Read the model definition and answer for the solid it produces. Units are mm, in the model's axes. Face numbers are marked on the shaded views. A direction names the side the tool comes from. Round coordinates to 2 decimals unless told otherwise and drop trailing zeros. Write each loop counter-clockwise with the first axis right and the second up, starting at its lowest first coordinate (ties: lowest second). Pieces come first, ordered by that corner, then holes.
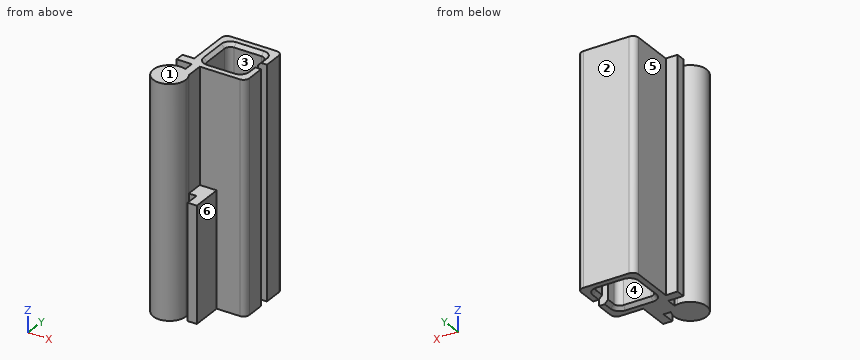
from build123d import *

# Parameters (mm, degrees)
F0_W     = 2.05
F0_H     = 1.6
F1_DEPTH = 40
F2_DEPTH = 20
F3_R     = 1
F4_SIZE  = 0.6


with BuildPart() as f1:
    # F0 (on Top) → F1 (new body)
    with BuildSketch(Plane.XY):
        Polygon((0.45, 6), (0.45, 4.4), (1.05, 4.4), (2.45, 4.4), (3.8, 4.4), (5.4, 4.4), (10.45, 4.4), (10.45, 8.6023478262), (8.85, 8.6023478262), (8.85, 6), (2.05, 6), (2.05, 12.8), (8.85, 12.8), (8.85, 10.1976521738), (10.45, 10.1976521738), (10.45, 14.4), (0.45, 14.4), align=None)
        with BuildLine():
            Line((2.45, 1.4), (2.45, 1.4560219779))
            ThreePointArc((2.45, 1.4560219779), (1.8489495156, 2.168844321), (1.05, 2.6495282599))
            Line((1.05, 2.6495282599), (0.45, 2.6495282599))
            Line((0.45, 2.6495282599), (0.45, 0))
            Line((0.45, 0), (2.45, 0))
            Line((2.45, 0), (2.45, 1.4))
        make_face()
        with BuildLine():
            ThreePointArc((0.45, 2.8142494559), (-2.1685248442, -1.8493242009), (2.85, 0))
            ThreePointArc((2.85, 0), (2.756578423, 0.723723288), (2.4824383175, 1.4))
            Line((2.4824383175, 1.4), (2.45, 1.4))
            Line((2.45, 1.4), (2.45, 0))
            Line((2.45, 0), (0.45, 0))
            Line((0.45, 0), (0.45, 2.6495282599))
            Line((0.45, 2.6495282599), (0.45, 2.8142494559))
        make_face()
        with BuildLine():
            ThreePointArc((1.05, 2.6495282599), (1.8489495156, 2.168844321), (2.45, 1.4560219779))
            Line((2.45, 1.4560219779), (2.45, 4.4))
            Line((2.45, 4.4), (1.05, 4.4))
            Line((1.05, 4.4), (1.05, 2.6495282599))
        make_face()
        with BuildLine():
            ThreePointArc((1.05, 2.6495282599), (0.7545086269, 2.7483116148), (0.45, 2.8142494559))
            Line((0.45, 2.8142494559), (0.45, 2.6495282599))
            Line((0.45, 2.6495282599), (1.05, 2.6495282599))
        make_face()
        with Locations((-0.575, 5.2)):
            Rectangle(F0_W, F0_H)
    extrude(amount=F1_DEPTH)

    # F0 (on Top) → F2 (join)
    with BuildSketch(Plane.XY):
        Polygon((3.8, 4.4), (3.8, 1.4), (3.8, -1), (5.4, -1), (5.4, 4.4), align=None)
        with BuildLine():
            Line((2.45, 1.4), (2.4824383175, 1.4))
            ThreePointArc((2.4824383175, 1.4), (2.4663782261, 1.4281030935), (2.45, 1.4560219779))
            Line((2.45, 1.4560219779), (2.45, 1.4))
        make_face()
        with BuildLine():
            ThreePointArc((2.45, 1.4560219779), (2.4663782261, 1.4281030935), (2.4824383175, 1.4))
            Line((2.4824383175, 1.4), (3.8, 1.4))
            Line((3.8, 1.4), (3.8, 4.4))
            Line((3.8, 4.4), (2.45, 4.4))
            Line((2.45, 4.4), (2.45, 1.4560219779))
        make_face()
    extrude(amount=F2_DEPTH)

    # F3
    f3_edges = [f1.edges().sort_by_distance(p)[0] for p in [
        (10.45, 14.4, 20),
        (0.45, 14.4, 20),
        (10.45, 4.4, 20),
        (2.05, 12.8, 20),
        (8.85, 12.8, 20),
        (8.85, 6, 20),
        (2.05, 6, 20),
    ]]
    fillet(f3_edges, radius=F3_R)

    # F4
    f4_edges = [f1.edges().sort_by_distance(p)[0] for p in [
        (2.05, 9.4, 40),
        (5.45, 6, 0),
    ]]
    chamfer(f4_edges, length=F4_SIZE)


solid = f1.part
Q1. Which of the six approach directions +Z, -Z, +X, -X, +Y, -Y give full straight-line access (tool end or side, diameter ignored) to the marked faces 4, 5 and 6?
Verdict:
face 4: +Z, -Z
face 5: +Z, -Z, -X, +Y
face 6: +Z, -Z, +X, -Y
Q2. Flat-ended cylindrical pins translate along their axes: pin 1 Ø3.5 at (y, z) = (10, 23.5) entering from -X; pin 2 Ø4 at (x, z) = (6, 27.5) entering from -Y; pin 3 Ø5 at (y, z) = (3.5, 11) entering from -X. Find the tip coordinate at first contact, or state that the pin passes through.
Verdict:
pin 1: stops at x = 0.45
pin 2: stops at y = 4.4
pin 3: stops at x = -2.67
Q3. Section C-C (x = 6.5) is taken. Determine the outline of the cut face in (y, z).
Verdict:
outline: (4.4, 0) - (5.4, 0) - (6, 0.6) - (6, 39.4) - (5.4, 40) - (4.4, 40) - close; (12.8, 0.6) - (13.4, 0) - (14.4, 0) - (14.4, 40) - (13.4, 40) - (12.8, 39.4) - close
Q4. Section D-D (z = 14.5) is taken. Determine the outline of the cut face in (x, y).
Verdict:
outline: (-1.6, 4.4) - (1.05, 4.4) - (1.05, 2.65) arc R2.85 ccw (long way) to (2.48, 1.4) - (3.8, 1.4) - (3.8, -1) - (5.4, -1) - (5.4, 4.4) - (9.45, 4.4) arc R1 ccw to (10.45, 5.4) - (10.45, 8.6) - (8.85, 8.6) - (8.85, 7) arc R1 cw to (7.85, 6) - (3.05, 6) arc R1 cw to (2.05, 7) - (2.05, 11.8) arc R1 cw to (3.05, 12.8) - (7.85, 12.8) arc R1 cw to (8.85, 11.8) - (8.85, 10.2) - (10.45, 10.2) - (10.45, 13.4) arc R1 ccw to (9.45, 14.4) - (1.45, 14.4) arc R1 ccw to (0.45, 13.4) - (0.45, 6) - (-1.6, 6) - close
Q5. Straight lines are drawn through the part: probe 1 along Y at (x, z) = (5, 21); probe 2 along X at (y, z) = (11, 32.5); probe 3 along Y at (x, z) = (9.5, 33). For each, find the intervals that lie inside material, in ascending order.
Verdict:
probe 1: y = 4.4 to 6, 12.8 to 14.4
probe 2: x = 0.45 to 2.05, 8.85 to 10.45
probe 3: y = 4.4 to 8.6, 10.2 to 14.4
Q6. Section A-A (x = 0) is taken. Determine the outline of the cut face in (y, z), then the cut area to 3 significant figures.
Verdict:
outline: (-2.85, 0) - (2.85, 0) - (2.85, 40) - (-2.85, 40) - close; (4.4, 0) - (6, 0) - (6, 40) - (4.4, 40) - close
area: 292 mm2
Q7. Determine the mould class of the marked faces 1, 2 and 3 for opening direction Y: pulls with the +Y half, pulls with the -Y half, needs draft (parallel to the pull), parting line crosses it, or undercut.
Verdict:
face 1: needs draft
face 2: pulls with the +Y half
face 3: undercut
